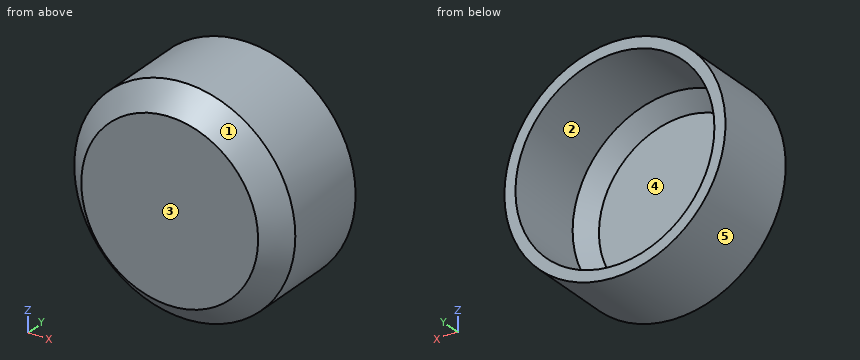
from build123d import *

# Parameters (mm, degrees)
F0_R     = 25.4
F1_DEPTH = 25.4
F2_SIZE  = 5.08
F3_T     = -2.54


with BuildPart() as f1:
    # F0 (on Front) → F1 (new body)
    with BuildSketch(Plane.XZ):
        Circle(F0_R)
    extrude(amount=F1_DEPTH)

    # F2
    f2_edges = [f1.edges().sort_by_distance(p)[0] for p in [
        (-25.4, -25.4, 0),
    ]]
    chamfer(f2_edges, length=F2_SIZE)

    # F3
    f3_openings = [f1.faces().sort_by_distance(p)[0] for p in [
        (0, 0, 0),
    ]]
    offset(amount=F3_T, openings=f3_openings)


solid = f1.part
The model under review builds one solid part; all positions refer to its coordinate system, in mm. Face numbers are marked on the shaded views. A direction names the side the tool comes from. Round coordinates to 2 decimals unless told otherwise and drop trailing zeros. Loops run counter-clockwise (first coordinate to the right, second up) from the corner with the lowest first, then second, coordinate; pieces in that order, holes last. Notation, with made-up numbers: (38, -24) -> (89, -24) arc R35 ccw to (89, 15) -> close; hole circle Ø3 at (11, -20.75). An arc over 180 degrees is marked (long way). Return JSON: item names as keys, results as strings.
(1) For pin 1 (2 mm diameter, centred on y = -21, z = 3.5, fed in from -X); pin 2 (5 mm diameter, centred on x = -5, z = 9, fed in from +Y); pin 3 (1 mm diameter, centred on x = -5.5, y = -18, fed in from -Z), all flat-tipped, find the tip position at first contact; note any pin that passes through.
Solved:
{"pin 1": "x = -25.25", "pin 2": "y = -22.86", "pin 3": "z = -24.9"}
(2) For line 1 (Z direction, x = 0, y = -11.5); line 2 (Y direction, x = -5.5, z = 0); line 3 (Z direction, x = -9, y = -10), list the stretches that pass through material, from the lowest coordinate up.
Solved:
{"line 1": "-25.4 to -22.86, 22.86 to 25.4", "line 2": "-25.4 to -22.86", "line 3": "-23.75 to -21.01, 21.01 to 23.75"}
(3) Add section A-A on y = -2.75. Write out the cut boundary in (x, z), plus the area to 3 significant figures.
Solved:
{"outline": "circle Ø50.8 at (0, 0); hole circle Ø45.72 at (0, 0)", "area": "385 mm2"}
(4) For the marked faces 1 and 2, list the 3-axis set-ups (+Z, -Z, +X, -X, +Y, -Y) from which the entire face can be reached by the end or side of a thin tool; tool diameter is ignored.
Solved:
{"face 1": "-Y", "face 2": "+Y"}
(5) Add section C-C on y = -21. Write out the cut boundary in (x, z), plus the area to 3 significant figures.
Solved:
{"outline": "circle Ø49.44 at (0, 0); hole circle Ø42.26 at (0, 0)", "area": "517 mm2"}
(6) The part is to be moulded in two halves that separate along Z. For the marked faces 3, 4 and 5, say which applies: released by +Z, released by -Z, zero draft, split by the parting line, or undercut.
Solved:
{"face 3": "zero draft", "face 4": "undercut", "face 5": "split by the parting line"}
(7) Add section B-B on z = 0. Write out the cut boundary in (x, y), plus the area to 3 significant figures.
Solved:
{"outline": "(-25.4, -20.32) -> (-20.32, -25.4) -> (20.32, -25.4) -> (25.4, -20.32) -> (25.4, 0) -> (22.86, 0) -> (22.86, -19.27) -> (19.27, -22.86) -> (-19.27, -22.86) -> (-22.86, -19.27) -> (-22.86, 0) -> (-25.4, 0) -> close", "area": "232 mm2"}
